Autodesk Inventor part; units mm, degrees
ref_plane "YZ Plane" through (0, 0, 0) normal (1, 0, 0) x (0, 1, 0)
ref_plane "XZ Plane" through (0, 0, 0) normal (0, 1, 0) x (-1, 0, 0)
ref_plane "XY Plane" through (0, 0, 0) normal (0, 0, 1) x (1, 0, 0)
sketch "Sketch1" plane through (0, 0, 0) normal (0, 1, 0) x (-1, 0, 0)
  line L0 (0, 0) -> (0, -31.748)
  line L1 (0, -31.748) -> (7.62, -31.748)
  line L2 (7.62, -31.748) -> (7.62, -26.16)
  line L3 (7.62, -26.16) -> (4.953, -26.16)
  line L4 (4.953, -26.16) -> (4.953, -23.493)
  line L5 (4.953, -23.493) -> (7.62, -23.493)
  line L6 (7.62, -23.493) -> (7.62, -17.016)
  line L7 (7.62, -17.016) -> (2.54, -17.016)
  line L8 (2.54, -17.016) -> (2.54, 0)
  line L9 (0, 0) -> (2.54, 0)
  dimension "d0" = 31.748
  dimension "d1" = 7.62
  dimension "d2" = 5.588
  dimension "d3" = 2.667
  dimension "d4" = 2.667
  dimension "d5" = 6.477
  dimension "d6" = 5.08
  dimension "d7" = 2.54
revolve "Revolution1" add sketch "Sketch1" angle 360 about axis through (0, 0, 0) along (-1, 0, 0)
sketch "Sketch2" plane through (-7.62, 0, 0) normal (-1, 0, 0) x (0, 0, 1)
  circle A0 centre (28.954, 0) radius 1.5
  circle A1 centre (0, 0) radius 31.748
  line L0 (31.748, 0) -> (26.16, 0)
  circle A2 centre (0, 0) radius 26.16
  circle A3 centre (0, 28.954) radius 1.5
  circle A4 centre (-28.954, 0) radius 1.5
  circle A5 centre (0, -28.954) radius 1.5
  dimension "d9" = 3
  dimension "d12" = 360
extrude "Extrusion1" cut sketch "Sketch2" against normal blind 12.7 contours L0 A0 | A0 L0 | A3 | A4 | A5
sketch "Sketch3" plane through (0, 0, 0) normal (1, 0, 0) x (0, 0, -1)
  circle A0 centre (0, 0) radius 23.493
  circle A1 centre (0, 0) radius 20.2545
  circle A2 centre (20.2545, 0) radius 1.5
  circle A3 centre (0, 20.2545) radius 1.5
  circle A4 centre (-20.2545, 0) radius 1.5
  circle A5 centre (0, -20.2545) radius 1.5
  dimension "d17" = 3.2385
  dimension "d18" = 3
  dimension "d21" = 360
sketch "Sketch4" plane through (-7.62, 0, 0) normal (-1, 0, 0) x (0, 0, 1)
  circle A0 centre (0, 0) radius 17.016
  circle A1 centre (0, 0) radius 23.493
  dimension "d16" = 6.477
extrude "Extrusion2" cut sketch "Sketch3" against normal blind 5.08 contours A1 A2 | A1 A2 | A3 A1 | A1 A3 | A5 A1 | A1 A5 | A4 A1 | A1 A4
sketch "Sketch5" plane through (-2.54, 0, 0) normal (-1, 0, 0) x (0, 0, 1)
  circle A0 centre (0, 0) radius 17.016
  line L0 (-17.016, 0) -> (17.016, 0)
  line L1 (-14.478, -9.9949) -> (14.478, -9.9949)
  line L2 (-14.478, 9.9949) -> (14.478, 9.9949)
  line L3 (14.478, 9.9949) -> (14.478, -9.9949)
  line L4 (-14.478, 9.9949) -> (-14.478, -9.9949)
  arc A1 (16.8267, -2.5309) -> (16.8267, 2.5309) centre (0, 0) ccw
  point P0 (0, 9.9949)
  point P1 (14.478, 0)
  dimension "d25" = 28.956
  dimension "d26" = 19.9898
sketch "Sketch6" plane through (-7.62, 0, 0) normal (-1, 0, 0) x (0, 0, 1)
  circle A0 centre (0, 0) radius 17.016
  circle A1 centre (17.016, 0) radius 2.54
  arc A2 (16.8264, -2.5329) -> (16.8264, 2.5329) centre (0, 0) ccw
  circle A3 centre (-17.016, -0.0173) radius 2.54
  arc A4 (-16.829, 2.5158) -> (-16.8238, -2.55) centre (0, 0) ccw
  dimension "d27" = 5.08
  dimension "d28" = 5.08
extrude "Extrusion3" cut sketch "Sketch6" against normal blind 12.7 contours A0 A1 | A3 A0 picked at (16.1885, -0.4913) picked at (-16.1553, -0.0173)
sketch "Sketch7" plane through (-2.54, 0, 17.016) normal (-1, 0, 0) x (0, 0, 1)
  circle A0 centre (-25.6012, 5.588) radius 1.8288
  circle A1 centre (-8.4308, 5.588) radius 1.8288
  arc A2 (-33.8398, -2.55) -> (-33.8449, 2.5158) centre (-34.0319, -0.0173) ccw
  line L0 (-31.4919, -0.0173) -> (-2.4894, -0.0173) construction
  line L1 (-25.6012, 5.588) -> (-8.4308, 5.588)
  circle A3 centre (-25.6012, 5.588) radius 1.8288
  circle A4 centre (-8.4308, 5.588) radius 1.8288
  point P0 (-17.016, 0)
  point P1 (-17.016, 5.588)
  dimension "d31" = 3.6576
  dimension "d32" = 3.6576
  dimension "d33" = 13.5128
  dimension "d34" = 5.588
equation "\"d28\" = d27"
equation "\"d32\" = d31"
Build history of the part. All positions in model axes, mm. A direction names the side the tool comes from. Round coordinates to 2 decimals unless told otherwise and drop trailing zeros. Loops run counter-clockwise (first coordinate to the right, second up) from the corner with the lowest first, then second, coordinate; pieces in that order, holes last. Notation, with made-up numbers: (-8.75, 11.5) -> (15.25, 11.5) arc R14 ccw to (15.25, 28.5) -> close; hole circle Ø8 at (-13, 56). An arc over 180 degrees is marked (long way). Use CSV: the item, a comma, the result in double quotes. Start each with the question number.
Q1. Flat gauge pins, fed straight in: pin 1 Ø2.5 at (y, z) = (0, -28.954) entering from +X; pin 2 Ø3 at (x, y) = (-5.5, 6.5) entering from -Z; pin 3 Ø4 at (x, z) = (-6, -19) entering from -Y; pin 4 Ø1.5 at (x, z) = (-3, 25) entering from -Y. Where does each tip first touch, or does it go through?
Q2. Mould opens along Z. For faces 6 (the face through (-3.863, -1.396, 31.717)), 7 (the face through (-2.504, 0.066, -18.756)), 8 (the face through (-7.62, -7, -16)) say: +Z half, -Z half, draft (parallel to the pull), parting line (faces both ways), or undercut.
Q3. Which spindle directions (+Z, -Z, +X, -X, +Y, -Y) get a long thin tool onto all of the face, cutting with end or side? Do faces 1 (the face through (-6.31, 14.3, 18.64)), 2 (the face through (-7.62, -12, 24)), 3 (the face through (-5.08, 20, 0)), 4 (the face through (0, 0, 0)), 5 (the face through (-1.288, 0.018, -17.016)). Say none if no direction does.
Q4. Saw through at C-C on y = -10. Give the cut face in (x, z).
Q5. Saw through at D-D on z = 7. Give the cut face in (x, y).
Q6. Drill centre lines: L1, parallel to Y at x = -5.95, z = 0; L2, parallel to Y at x = -3, z = 0; L3, parallel to Z at x = -6.75, y = -14. Where is each one in solid material? Low to high.
Q7. Saw through at A-A on z = 0. Count the separate pieces of the cut face and the enclosed holes in it, and give its area (3 significant figures).
Solutions:
1,pin 1,"passes through"
1,pin 2,"stops at z = -31.35"
1,pin 3,"stops at y = -26.81"
1,pin 4,"stops at y = -20.49"
2,face 6,"parting line"
2,face 7,"undercut"
2,face 8,"draft"
3,face 1,"-X"
3,face 2,"+Z, -Z, -X, +Y, -Y"
3,face 3,"+X"
3,face 4,"+Z, -Z, +X, +Y, -Y"
3,face 5,"+X, -X"
4,outline,"(-7.62, -30.13) -> (0, -30.13) -> (0, 30.13) -> (-7.62, 30.13) -> (-7.62, 24.17) -> (-4.95, 24.17) -> (-4.95, 21.26) -> (-7.62, 21.26) -> (-7.62, 13.77) -> (-2.54, 13.77) -> (-2.54, -13.77) -> (-7.62, -13.77) -> (-7.62, -21.26) -> (-4.95, -21.26) -> (-4.95, -24.17) -> (-7.62, -24.17) -> close"
5,outline,"(-7.62, -30.97) -> (0, -30.97) -> (0, 30.97) -> (-7.62, 30.97) -> (-7.62, 25.21) -> (-4.95, 25.21) -> (-4.95, 22.43) -> (-7.62, 22.43) -> (-7.62, 15.51) -> (-2.54, 15.51) -> (-2.54, -15.51) -> (-7.62, -15.51) -> (-7.62, -22.43) -> (-4.95, -22.43) -> (-4.95, -25.21) -> (-7.62, -25.21) -> close"
6,L1,"y = -31.75 to -30.45, -27.45 to -26.16, -23.49 to -17.02, 17.02 to 23.49, 26.16 to 27.45, 30.45 to 31.75"
6,L2,"y = -31.75 to -30.45, -27.45 to -21.75, -18.75 to -17.02, 17.02 to 18.75, 21.75 to 27.45, 30.45 to 31.75"
6,L3,"z = -28.49 to -22.1, -18.87 to -9.67, 9.67 to 18.87, 22.1 to 28.49"
7,separate pieces,"3"
7,enclosed holes,"0"
7,area,"221 mm^2"
